Design review of the part built by this model. Coordinates are the model's own, in mm. A direction names the side the tool comes from. Round coordinates to 2 decimals unless told otherwise and drop trailing zeros. Order: outer loops, then holes, each group sorted by start corner. A loop starts at its lowest first (then second) coordinate and runs counter-clockwise, first axis right, second up. Notation, with made-up numbers: M 14,-14.5 L 69,-14.5 A18 cw 69,9.5 Z; hole C -9,-35.5 d1. An arc over 180 degrees is marked long. Use a Markdown table: item, result. Add a question column.
(1) Machinability: for faces 3 (the face through (2, -5, 0)), 4 (the face through (51.89, 105.35, 1.52)), which of the approach directions +Z, -Z, +X, -X, +Y, -Y give a long, thin tool a straight path to every point of the face, cutting with its end or side? Answer none if there is none.
(2) To check wall thickness, follow probe 1 along Y at (x, z) = (-21, 1.45); probe 2 along Y at (x, z) = (-4.5, 2.85); probe 3 along X at (y, z) = (33, 1.5). State the ranges of each line that lie inside material, in increasing order. Write a range as from..to.
(3) Take a section at C-C (x = 107). Write out the cut boundary in (y, z).
(4) For pin 1 (3 mm diameter, centred on x = 51.5, y = 30, fed in from +Z); pin 2 (1.5 mm diameter, centred on y = -82.5, z = 2, fed in from +X); pin 3 (0.9 mm diameter, centred on y = -80.5, z = 1, fed in from -X); pin 4 (0.9 mm diameter, centred on y = -81, z = 2, fed in from -X), all flat-tipped, find the tip position at first contact; note any pin that passes through.
(5) Take a section at B-B (y = 42). Write out the cut boundary in (x, z), then the cut area to 3 significant figures.
(6) The part is to be moulded in two halves that separate along Y. For faces 1 (the face through (-51.89, 105.35, 1.52)), 2 (the face through (2, -5, 3)), say which applies: released by +Y, released by -Y, zero draft, split by the parting line, or undercut.
(7) Take a section at A-A (x = 35.5). Write out the cut boundary in (y, z), then the cut area to 3 significant figures.
(8) Take a section at D-D (y = -20.5). Write out the cut boundary in (x, z).
```python
from build123d import *

# Parameters (mm, degrees)
BOSS_EXTRUDE1_DEPTH  = 3
CUT_EXTRUDE2_START   = -3
CUT_EXTRUDE2_DEPTH   = 208.044112878
LPATTERN2_COUNT      = 8
LPATTERN2_PITCH      = 25
MIRROR1_START        = -3
MIRROR1_COPY_1_DEPTH = 208.044112878
MIRROR1_COPY_2_DEPTH = 208.044112878
MIRROR1_COPY_3_DEPTH = 208.044112878
MIRROR1_COPY_4_DEPTH = 208.044112878
MIRROR1_COPY_5_DEPTH = 208.044112878
MIRROR1_COPY_6_DEPTH = 208.044112878
MIRROR1_COPY_7_DEPTH = 208.044112878
CUT_EXTRUDE3_START   = -3
CUT_EXTRUDE3_DEPTH   = 208.044112878
LPATTERN3_COUNT      = 2
LPATTERN3_PITCH      = 25
MIRROR2_START        = -3
MIRROR2_COPY_1_DEPTH = 208.044112878
SKETCH5_W            = 10
SKETCH5_H            = 10
CUT_EXTRUDE7_DEPTH   = 10
LPATTERN5_COUNT      = 15
LPATTERN5_PITCH      = 21
SKETCH9_W            = 109.8
SKETCH9_H            = 11.8
BOSS_EXTRUDE2_DEPTH  = 3
FILLET1_R            = 10


with BuildPart() as part:
    # Sketch1 → Boss-Extrude1 (new body)
    with BuildSketch(Plane.XY):
        Polygon((-111.410161514, 120), (-54.9, 120), (-54.9, 0), (54.9, 0), (54.9, 120), (111.410161514, 120), (114.865412578, 106.649935044), (117.371040649, 96.968931585), (165, -87.055236082), (-165, -87.055236082), align=None)
    extrude(amount=BOSS_EXTRUDE1_DEPTH)

    # Sketch3 → Cut-Extrude2 (cut)
    with BuildSketch(Plane.XY.offset(3).offset(CUT_EXTRUDE2_START)):
        Polygon((117.674231691, 95.797491353), (115.16860362, 105.478494812), (112.264302582, 104.72680639), (114.769930653, 95.045802932), align=None)
    cut_extrude2 = extrude(amount=CUT_EXTRUDE2_DEPTH, mode=Mode.SUBTRACT)

    # LPattern2: Cut-Extrude2 ×8
    with Locations(*[Vector(0.2505628070857313, -0.968100345886375, 0) * (i * LPATTERN2_PITCH) for i in range(1, LPATTERN2_COUNT)]):
        add(cut_extrude2, mode=Mode.SUBTRACT)

    # Mirror1: Cut-Extrude2 across plane
    add(cut_extrude2.mirror(Plane(origin=(0, 0, 0), x_dir=(0, 0, 1), z_dir=(1, 0, 0))), mode=Mode.SUBTRACT)

    # Mirror1 copy 1 sketch → Mirror1 copy 1 (cut)
    with BuildSketch(Plane(origin=(-6.264070177, -24.202508647, 3), x_dir=(-1, 0, 0), z_dir=(0, 0, 1)).offset(MIRROR1_START)):
        Polygon((117.674231691, -95.797491353), (115.16860362, -105.478494812), (112.264302582, -104.72680639), (114.769930653, -95.045802932), align=None)
    extrude(amount=MIRROR1_COPY_1_DEPTH, mode=Mode.SUBTRACT)

    # Mirror1 copy 2 sketch → Mirror1 copy 2 (cut)
    with BuildSketch(Plane(origin=(-12.528140354, -48.405017294, 3), x_dir=(-1, 0, 0), z_dir=(0, 0, 1)).offset(MIRROR1_START)):
        Polygon((117.674231691, -95.797491353), (115.16860362, -105.478494812), (112.264302582, -104.72680639), (114.769930653, -95.045802932), align=None)
    extrude(amount=MIRROR1_COPY_2_DEPTH, mode=Mode.SUBTRACT)

    # Mirror1 copy 3 sketch → Mirror1 copy 3 (cut)
    with BuildSketch(Plane(origin=(-18.792210531, -72.607525941, 3), x_dir=(-1, 0, 0), z_dir=(0, 0, 1)).offset(MIRROR1_START)):
        Polygon((117.674231691, -95.797491353), (115.16860362, -105.478494812), (112.264302582, -104.72680639), (114.769930653, -95.045802932), align=None)
    extrude(amount=MIRROR1_COPY_3_DEPTH, mode=Mode.SUBTRACT)

    # Mirror1 copy 4 sketch → Mirror1 copy 4 (cut)
    with BuildSketch(Plane(origin=(-25.056280709, -96.810034589, 3), x_dir=(-1, 0, 0), z_dir=(0, 0, 1)).offset(MIRROR1_START)):
        Polygon((117.674231691, -95.797491353), (115.16860362, -105.478494812), (112.264302582, -104.72680639), (114.769930653, -95.045802932), align=None)
    extrude(amount=MIRROR1_COPY_4_DEPTH, mode=Mode.SUBTRACT)

    # Mirror1 copy 5 sketch → Mirror1 copy 5 (cut)
    with BuildSketch(Plane(origin=(-31.320350886, -121.012543236, 3), x_dir=(-1, 0, 0), z_dir=(0, 0, 1)).offset(MIRROR1_START)):
        Polygon((117.674231691, -95.797491353), (115.16860362, -105.478494812), (112.264302582, -104.72680639), (114.769930653, -95.045802932), align=None)
    extrude(amount=MIRROR1_COPY_5_DEPTH, mode=Mode.SUBTRACT)

    # Mirror1 copy 6 sketch → Mirror1 copy 6 (cut)
    with BuildSketch(Plane(origin=(-37.584421063, -145.215051883, 3), x_dir=(-1, 0, 0), z_dir=(0, 0, 1)).offset(MIRROR1_START)):
        Polygon((117.674231691, -95.797491353), (115.16860362, -105.478494812), (112.264302582, -104.72680639), (114.769930653, -95.045802932), align=None)
    extrude(amount=MIRROR1_COPY_6_DEPTH, mode=Mode.SUBTRACT)

    # Mirror1 copy 7 sketch → Mirror1 copy 7 (cut)
    with BuildSketch(Plane(origin=(-43.84849124, -169.41756053, 3), x_dir=(-1, 0, 0), z_dir=(0, 0, 1)).offset(MIRROR1_START)):
        Polygon((117.674231691, -95.797491353), (115.16860362, -105.478494812), (112.264302582, -104.72680639), (114.769930653, -95.045802932), align=None)
    extrude(amount=MIRROR1_COPY_7_DEPTH, mode=Mode.SUBTRACT)

    # Sketch4 → Cut-Extrude3 (cut)
    with BuildSketch(Plane.XY.offset(3).offset(CUT_EXTRUDE3_START)):
        Polygon((-96.410161514, 796.954701105), (-96.410161514, 120), (-96.410161514, 117), (-86.410161514, 117), (-86.410161514, 120), (-86.410161514, 796.954701105), (-86.410161514, 2150.864103316), (-96.410161514, 2150.864103316), align=None)
    cut_extrude3 = extrude(amount=CUT_EXTRUDE3_DEPTH, mode=Mode.SUBTRACT)

    # LPattern3: Cut-Extrude3 ×2
    with Locations(*[(i * LPATTERN3_PITCH, 0, 0) for i in range(1, LPATTERN3_COUNT)]):
        add(cut_extrude3, mode=Mode.SUBTRACT)

    # Mirror2: Cut-Extrude3 across plane
    add(cut_extrude3.mirror(Plane(origin=(0, 0, 0), x_dir=(0, 0, 1), z_dir=(1, 0, 0))), mode=Mode.SUBTRACT)

    # Mirror2 copy 1 sketch → Mirror2 copy 1 (cut)
    with BuildSketch(Plane(origin=(-25, 0, 3), x_dir=(-1, 0, 0), z_dir=(0, 0, 1)).offset(MIRROR2_START)):
        Polygon((-96.410161514, -796.954701105), (-96.410161514, -120), (-96.410161514, -117), (-86.410161514, -117), (-86.410161514, -120), (-86.410161514, -796.954701105), (-86.410161514, -2150.864103316), (-96.410161514, -2150.864103316), align=None)
    extrude(amount=MIRROR2_COPY_1_DEPTH, mode=Mode.SUBTRACT)

    # Sketch5 → Cut-Extrude7 (cut)
    with BuildSketch(Plane.XY.offset(3)):
        with Locations((-145, -82.055236082)):
            Rectangle(SKETCH5_W, SKETCH5_H)
    cut_extrude7 = extrude(amount=-CUT_EXTRUDE7_DEPTH, mode=Mode.SUBTRACT)

    # LPattern5: Cut-Extrude7 ×15
    with Locations(*[(i * LPATTERN5_PITCH, 0, 0) for i in range(1, LPATTERN5_COUNT)]):
        add(cut_extrude7, mode=Mode.SUBTRACT)

    # Sketch9 → Boss-Extrude2 (add)
    with BuildSketch(Plane(origin=(0, 0, 0), x_dir=(-1, 0, 0), z_dir=(0, 0, -1))):
        with Locations((0, 114.1)):
            Rectangle(SKETCH9_W, SKETCH9_H)
    extrude(amount=-BOSS_EXTRUDE2_DEPTH)

    # Fillet1
    fillet1_edges = [part.edges().sort_by_distance(p)[0] for p in [
        (54.9, 108.2, 1.5),
        (-54.9, 108.2, 1.5),
    ]]
    fillet(fillet1_edges, radius=FILLET1_R)


solid = part.part
```
Verdict:
| question | item | result |
|---|---|---|
| 1 | face 3 | -Z, +X, -X, +Y, -Y |
| 1 | face 4 | +Z, -Z |
| 2 | probe 1 | y = -77.06..0, 108.2..120 |
| 2 | probe 2 | y = -87.06..0, 108.2..120 |
| 2 | probe 3 | x = -133.93..-54.9, 54.9..133.93 |
| 3 | outline | M -77.06,0 L 120,0 L 120,3 L -77.06,3 Z |
| 4 | pin 1 | passes through |
| 4 | pin 2 | stops at x = 164.02 |
| 4 | pin 3 | stops at x = -163.42 |
| 4 | pin 4 | stops at x = -163.55 |
| 5 | outline | M -131.6,0 L -54.9,0 L -54.9,3 L -131.6,3 Z; M 54.9,0 L 131.6,0 L 131.6,3 L 54.9,3 Z |
| 5 | area | 460 mm^2 |
| 6 | face 1 | undercut |
| 6 | face 2 | zero draft |
| 7 | outline | M -87.06,0 L 0,0 L 0,3 L -87.06,3 Z; M 108.2,0 L 120,0 L 120,3 L 108.2,3 Z |
| 7 | area | 297 mm^2 |
| 8 | outline | M -144.68,0 L 144.68,0 L 144.68,3 L -144.68,3 Z |
